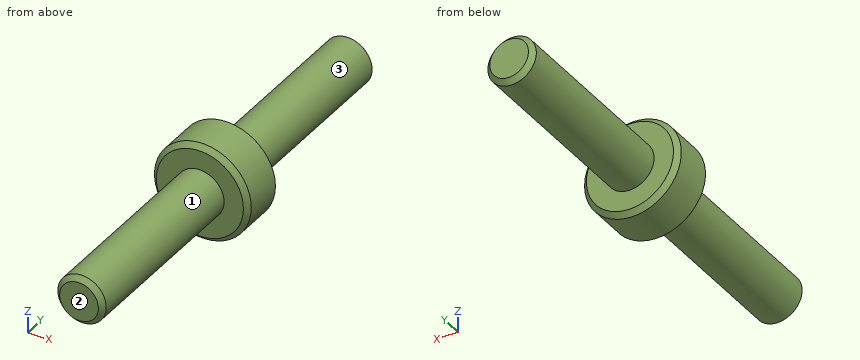
from build123d import *

# Parameters (mm, degrees)
F0_R     = 3.175
F1_DEPTH = 28.575
F0_R_2   = 6.35
F2_DEPTH = 3.175
F3_SIZE  = 0.635


with BuildPart() as f1:
    # F0 (on Front) → F1 (new body, symmetric)
    with BuildSketch(Plane.XZ):
        Circle(F0_R)
    extrude(amount=F1_DEPTH, both=True)

    # F0 (on Front) → F2 (join, symmetric)
    with BuildSketch(Plane.XZ):
        Circle(F0_R_2)
        Circle(F0_R, mode=Mode.SUBTRACT)
    extrude(amount=F2_DEPTH, both=True)

    # F3
    f3_edges = [f1.edges().sort_by_distance(p)[0] for p in [
        (-3.175, -28.575, 0),
        (-3.175, 28.575, 0),
        (-6.35, -3.175, 0),
        (-6.35, 3.175, 0),
    ]]
    chamfer(f3_edges, length=F3_SIZE)


solid = f1.part
Geometry: final body of the model. Coordinates: model frame, mm. Face numbers are marked on the shaded views. A direction names the side the tool comes from. Coordinates: 2 decimals unless noted, no trailing zeros. Order: outer loops, then holes, each group sorted by start corner. A loop starts at its lowest first (then second) coordinate and runs counter-clockwise, first axis right, second up.
1) Section D-D (y = 9). Return loops of the section in (x, z) (3 decimals).
Result sheet:
outline: circle Ø6.35 at (0, 0)
2) Ray query, probe 1 along Y at (x, z) = (4.5, -2.75) (3 decimals); probe 2 along X at (y, z) = (20, -0.25); probe 3 along Z at (x, y) = (-2.75, 18). Return the intervals inside material, ascending.
Result sheet:
probe 1: y = -3.175 to 3.175
probe 2: x = -3.17 to 3.17
probe 3: z = -1.59 to 1.59
3) Section C-C (y = 2). Return loops of the section in (x, z), then the cut area to 3 significant figures.
Result sheet:
outline: circle Ø12.7 at (0, 0)
area: 127 mm2
4) Section B-B (x = 0). Return loops of the section in (y, z) (3 decimals).
Result sheet:
outline: (-28.575, -2.54) - (-27.94, -3.175) - (-3.175, -3.175) - (-3.175, -5.715) - (-2.54, -6.35) - (2.54, -6.35) - (3.175, -5.715) - (3.175, -3.175) - (27.94, -3.175) - (28.575, -2.54) - (28.575, 2.54) - (27.94, 3.175) - (3.175, 3.175) - (3.175, 5.715) - (2.54, 6.35) - (-2.54, 6.35) - (-3.175, 5.715) - (-3.175, 3.175) - (-27.94, 3.175) - (-28.575, 2.54) - close
5) Section A-A (z = 0). Return loops of the section in (x, y) (3 decimals).
Result sheet:
outline: (-6.35, -2.54) - (-5.715, -3.175) - (-3.175, -3.175) - (-3.175, -27.94) - (-2.54, -28.575) - (2.54, -28.575) - (3.175, -27.94) - (3.175, -3.175) - (5.715, -3.175) - (6.35, -2.54) - (6.35, 2.54) - (5.715, 3.175) - (3.175, 3.175) - (3.175, 27.94) - (2.54, 28.575) - (-2.54, 28.575) - (-3.175, 27.94) - (-3.175, 3.175) - (-5.715, 3.175) - (-6.35, 2.54) - close
6) First-contact query: P1, Ø5, axis at x = 1.5, y = -13, coming from the +Z side (3 decimals); P2, Ø1.5, axis at x = -2.5, y = -4.5, coming from the -Z side. Flat tips, straight axial feed; report the tip coordinate or a pass-through.
Result sheet:
P1: stops at z = 3.175
P2: stops at z = -2.65
7) Set-up query: the marked faces 1, 2 and 3. Return all of +Z, -Z, +X, -X, +Y, -Y with unobstructed straight access to the full face (end or side cutting, diameter ignored); none if empty.
Result sheet:
face 1: -Y
face 2: +Z, -Z, +X, -X, -Y
face 3: +Y
